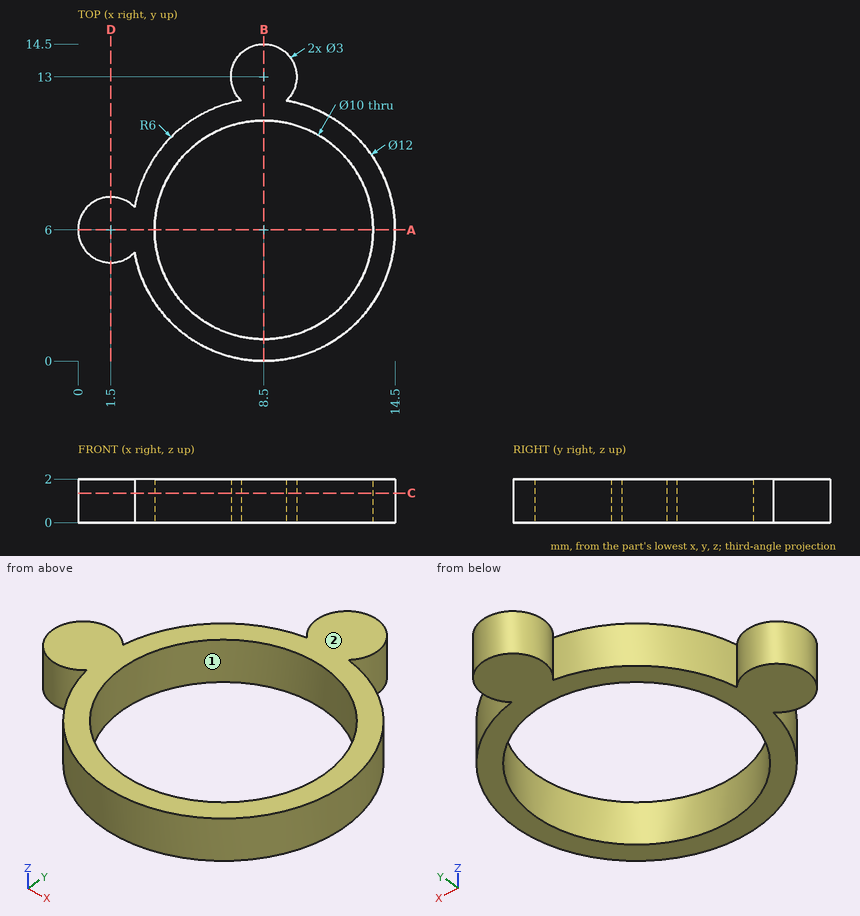
The figure shows three views and two pictorial views of one solid part (mm, origin at its lowest corner). Answer the questions. Give positions to 0.01 mm unless a question says otherwise; leave off trailing zeros. Order: outer loops, then holes, each group sorted by start corner. A loop starts at its lowest first (then second) coordinate and runs counter-clockwise, first axis right, second up. Notation, with made-up numbers: M -28,-23.5 L -6,-23.5 A21 ccw -6,8.5 Z; hole C -31,42 d8. An arc over 180 degrees is marked long. Return JSON: item names as keys, results as strings.
Q1. Find section A-A, the plane y = 6. Write down the section's boundary in (x, z).
Answer below:
{"outline": "M 0,0 L 3.5,0 L 3.5,2 L 0,2 Z; M 13.5,0 L 14.5,0 L 14.5,2 L 13.5,2 Z"}
Q2. Find section C-C, the plane z = 1.35. Write down the section's boundary in (x, y), and give its area (3 significant figures).
Answer below:
{"outline": "M 2.59,4.97 A6 ccw long 9.53,11.91 A1.5 ccw long 7.47,11.91 A6 ccw 2.59,7.03 A1.5 ccw long Z; hole C 8.5,6 d10", "area": "47.3 mm^2"}
Q3. Find section B-B, the plane x = 8.5. Write down the section's boundary in (y, z).
Answer below:
{"outline": "M 0,0 L 1,0 L 1,2 L 0,2 Z; M 11,0 L 14.5,0 L 14.5,2 L 11,2 Z"}
Q4. Find the intervals of material crossed by line 1 along Y through (x, z) = (8.5, 0.75); line 2 along Y through (x, z) = (7.5, 1.35); line 3 along X through (y, z) = (4.75, 1.95), in increasing order. Write a range as [from, to].
Answer below:
{"line 1": "y = [0, 1], [11, 14.5]", "line 2": "y = [0.08, 1.1], [10.9, 14.12]", "line 3": "x = [0.67, 2.33], [2.63, 3.66], [13.34, 14.37]"}
Q5. Find section D-D, the plane x = 1.5. Write down the section's boundary in (y, z).
Answer below:
{"outline": "M 4.5,0 L 7.5,0 L 7.5,2 L 4.5,2 Z"}
Q6. The mould has two halves that part along X. Classify the marked faces 1 and 2: pulls with the +X half, pulls with the -X half, needs draft (parallel to the pull), parting line crosses it, or undercut.
Answer below:
{"face 1": "undercut", "face 2": "needs draft"}
